from build123d import *

# Parameters (mm, degrees)
SKETCH1_W           = 88.168408076
SKETCH1_H           = 59.84281091
BOSS_EXTRUDE4_DEPTH = 2
SKETCH2_W           = 2
SKETCH2_H           = 59.84281091
BOSS_EXTRUDE5_DEPTH = 30
SKETCH3_W           = 84.168408076
SKETCH3_H           = 2
BOSS_EXTRUDE6_DEPTH = 30
SKETCH4_W           = 30
SKETCH4_H           = 38.84281091
CUT_EXTRUDE1_DEPTH  = 30
SKETCH5_W           = 2
SKETCH5_H           = 38.84281091
BOSS_EXTRUDE7_DEPTH = 86.168408075
SKETCH6_W           = 28
SKETCH6_H           = 38.84281091
CUT_EXTRUDE2_DEPTH  = 97.665842233


with BuildPart() as part:
    # Sketch1 → Boss-Extrude4 (new body)
    with BuildSketch(Plane.XY):
        Rectangle(SKETCH1_W, SKETCH1_H)
    extrude(amount=BOSS_EXTRUDE4_DEPTH)

    # Sketch2 → Boss-Extrude5 (add)
    with BuildSketch(Plane.XY.offset(2)):
        with Locations((-43.084204038, 0)):
            Rectangle(SKETCH2_W, SKETCH2_H)
        with Locations((43.084204038, 0)):
            Rectangle(SKETCH2_W, SKETCH2_H)
    extrude(amount=BOSS_EXTRUDE5_DEPTH)

    # Sketch3 → Boss-Extrude6 (add)
    with BuildSketch(Plane.XY.offset(2)):
        with Locations((0, 28.921405455)):
            Rectangle(SKETCH3_W, SKETCH3_H)
        with Locations((0, -28.921405455)):
            Rectangle(SKETCH3_W, SKETCH3_H)
        with Locations((0, 11.921405455)):
            Rectangle(SKETCH3_W, SKETCH3_H)
    extrude(amount=BOSS_EXTRUDE6_DEPTH)

    # Sketch4 → Cut-Extrude1 (cut)
    with BuildSketch(Plane(origin=(-42.084204038, 0, 0), x_dir=(0, 0, -1), z_dir=(1, 0, 0))):
        with Locations((-17, -8.5)):
            Rectangle(SKETCH4_W, SKETCH4_H)
    extrude(amount=-CUT_EXTRUDE1_DEPTH, mode=Mode.SUBTRACT)

    # Sketch5 → Boss-Extrude7 (add)
    with BuildSketch(Plane.ZY.offset(-42.084204038)):
        with Locations((31, -8.5)):
            Rectangle(SKETCH5_W, SKETCH5_H)
    extrude(amount=BOSS_EXTRUDE7_DEPTH)

    # Sketch6 → Cut-Extrude2 (cut, through all)
    with BuildSketch(Plane.ZY.offset(-42.084204038)):
        with Locations((16, -8.5)):
            Rectangle(SKETCH6_W, SKETCH6_H)
    extrude(amount=-CUT_EXTRUDE2_DEPTH, mode=Mode.SUBTRACT)


solid = part.part
Build history of the part. All positions in model axes, mm. A direction names the side the tool comes from. Give positions to 0.01 mm unless a question says otherwise; leave off trailing zeros. Write each loop counter-clockwise with the first axis right and the second up, starting at its lowest first coordinate (ties: lowest second). Pieces come first, ordered by that corner, then holes. Notation, with made-up numbers: (8, 60) - (55, 60) arc R5 ccw to (55, 66) - close; hole circle Ø9 at (46, 77). An arc over 180 degrees is marked (long way). Use one line per item in the form item = value. Start each with the question number.
1. Two-plate mould, pull along X, no slides. Class faces 1 (the face through (-1, -29.921, 16)), 2 (the face through (-1, 12.921, 17)), 3 (the face through (-1, 21, 2)), 4 (the face through (44.084, 13, 12)): released by +X, released by -X, zero draft, split by the parting line, or undercut.
2. Band-saw the part on A-A on z = 21.5. Write the cut outline in (x, y), plus the area to 3 significant figures.
3. Probe line 1 (Y direction, x = -8, z = 5); line 2 (X direction, y = 17, z = 17.5); line 3 (Y direction, x = 20, z = 30.5). List the from-to ranges inside material, lowest first. Write a range as [from, to].
4. Band-saw the part on C-C on x = 14.5. Write the cut outline in (y, z), plus the area to 3 significant figures.
5. Drop a flat-ended pin along its axis: pin 1 Ø4.5 at (x, y) = (-19.5, 21) entering from +Z. Give the stop position or say it passes through.
6. Band-saw the part on B-B on y = 0.5. Write the cut outline in (x, z), plus the area to 3 significant figures.
7. 3-axis set-ups, long thin cutter, end or side, ignore diameter. For faces 5 (the face through (-1, 27.921, 17)), 6 (the face through (-1, 10.921, 16)), 7 (the face through (1, -7, 32)): which of +Z, -Z, +X, -X, +Y, -Y reach the whole face in a straight line?
8. Band-saw the part on D-D on y = 20. Write the cut outline in (x, z).
Conclusion:
q1.face_1 = zero draft
q1.face_2 = undercut
q1.face_3 = undercut
q1.face_4 = released by +X
q2.outline = (-44.08, -29.92) - (44.08, -29.92) - (44.08, -27.92) - (-44.08, -27.92) - close; (-44.08, 10.92) - (44.08, 10.92) - (44.08, 29.92) - (-44.08, 29.92) - close; hole (-42.08, 12.92) - (42.08, 12.92) - (42.08, 27.92) - (-42.08, 27.92) - close
q2.area = 589 mm²
q3.line_1 = [-29.92, -27.92], [10.92, 12.92], [27.92, 29.92]
q3.line_2 = [-44.08, -42.08], [42.08, 44.08]
q3.line_3 = [-29.92, 12.92], [27.92, 29.92]
q4.outline = (-29.92, 0) - (29.92, 0) - (29.92, 32) - (27.92, 32) - (27.92, 2) - (12.92, 2) - (12.92, 32) - (-29.92, 32) - close; hole (-27.92, 2) - (10.92, 2) - (10.92, 30) - (-27.92, 30) - close
q4.area = 377 mm²
q5.pin_1 = 2
q6.outline = (-44.08, 0) - (44.08, 0) - (44.08, 2) - (-44.08, 2) - close; (-44.08, 30) - (44.08, 30) - (44.08, 32) - (-44.08, 32) - close
q6.area = 353 mm²
q7.face_5 = +Z
q7.face_6 = +X, -X
q7.face_7 = +Z, +X, -X, +Y, -Y
q8.outline = (-44.08, 0) - (44.08, 0) - (44.08, 32) - (42.08, 32) - (42.08, 2) - (-42.08, 2) - (-42.08, 32) - (-44.08, 32) - close
